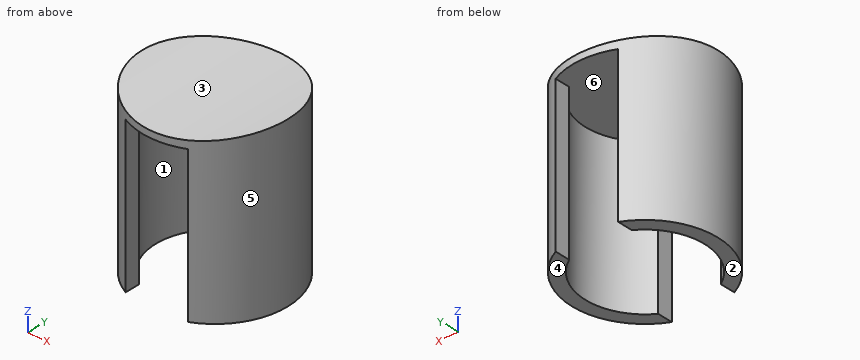
from build123d import *

# Parameters (mm, degrees)
F2_W     = 9.278574
F2_H     = 23.490808
F3_DEPTH = 22.747948
F4_R     = 65
F5_DEPTH = 12.5


with BuildPart() as f1:
    # F0 (on Front) → F1 (revolve)
    with BuildSketch(Plane.XZ):
        Polygon((10.8, -12.5), (10.8, 15.247948), (0, 15.247948), (0, 10.247948), (8.8, 10.247948), (8.8, -11.752052), (8.8, -12.5), align=None)
    revolve(axis=Axis((0, 0, 12.181249), (0, 0, 1)))

    # F2 (on face) → F3 (cut, through all)
    with BuildSketch(Plane(origin=(0, 0, -12.5), x_dir=(1, 0, 0), z_dir=(0, 0, -1))):
        Rectangle(F2_W, F2_H)
    extrude(amount=-F3_DEPTH, mode=Mode.SUBTRACT)

    # F4 (on Front) → F5 (cut, symmetric)
    with BuildSketch(Plane.XZ):
        with Locations((0, 76.247948)):
            Circle(F4_R)
    extrude(amount=F5_DEPTH, both=True, mode=Mode.SUBTRACT)


solid = f1.part
Can you work these out from the model? Positions are in its coordinate system, mm. Face numbers are marked on the shaded views. A direction names the side the tool comes from. Give positions to 0.01 mm unless a question says otherwise; leave off trailing zeros. Loops run counter-clockwise (first coordinate to the right, second up) from the corner with the lowest first, then second, coordinate; pieces in that order, holes last. Notation, with made-up numbers: (-16.75, 46.5) - (31.25, 46.5) arc R25 ccw to (31.25, 65.5) - close; hole circle Ø4 at (-27, 32). An arc over 180 degrees is marked (long way). One line per item, written item: value.
(1) If we section it at A-A, the plane z = -5: List the corners of the cut face in (x, y) for me.
Verdict:
outline: (-4.64, -9.75) - (-4.64, -7.48) arc R8.8 cw to (-4.64, 7.48) - (-4.64, 9.75) arc R10.8 ccw to start; (4.64, -9.75) arc R10.8 ccw to (4.64, 9.75) - (4.64, 7.48) arc R8.8 cw to (4.64, -7.48) - close
(2) If we section it at B-B, the plane y = 0: List the corners of the cut face in (x, z) for me.
Verdict:
outline: (-10.8, -12.5) - (-8.8, -12.5) - (-8.8, 10.25) - (8.8, 10.25) - (8.8, -12.5) - (10.8, -12.5) - (10.8, 12.15) arc R65 cw to (-10.8, 12.15) - close
(3) If we mould it in two halves opening along X, with no side actions, what happens to the marked faces 3, 4, 5 and 6? For each: released by +X, released by -X, zero draft, split by the parting line, or undercut.
Verdict:
face 3: undercut
face 4: zero draft
face 5: split by the parting line
face 6: undercut
(4) If we section it at C-C, the plane x = -5.5: List the corners of the cut face in (y, z) for me.
Verdict:
outline: (-9.29, -12.5) - (-6.87, -12.5) - (-6.87, 10.25) - (6.87, 10.25) - (6.87, -12.5) - (9.29, -12.5) - (9.29, 11.48) - (-9.29, 11.48) - close
(5) On a 3-axis mill with a long thin cutter (end or side, diameter ignored), from which of +Z, -Z, +X, -X, +Y, -Y can I reach the whole of each face in a straight line? I mean the marked faces 1 and 2. Say none if no direction works.
Verdict:
face 1: -Z
face 2: -Z, +X, -X, +Y, -Y
(6) I need wall thicknesses on line 1 along Z through (x, y) = (-1, -5.5); line 2 along X through (y, z) = (2.5, 4.5); line 3 along X through (y, z) = (-3, -1.75). Which ranges of each line are inside material? Lowest first, please.
Verdict:
line 1: 10.25 to 11.26
line 2: -10.51 to -8.44, 8.44 to 10.51
line 3: -10.37 to -8.27, 8.27 to 10.37
(7) I'm going to push flat-ended pins straight in: pin 1 (5.5 mm diameter, centred on x = 2.5, y = -5, fed in from -Z); pin 2 (6 mm diameter, centred on x = -8.5, z = -5.5, fed in from -Y); pin 3 (1.5 mm diameter, centred on x = -6.5, z = -3, fed in from +Y). Where does each tip first touch, or does it pass through?
Verdict:
pin 1: z = 10.25
pin 2: y = -9.29
pin 3: y = 9.14
(8) If we section it at D-D, the plane x = 0: List the corners of the cut face in (y, z) for me.
Verdict:
outline: (-10.8, 10.25) - (10.8, 10.25) - (10.8, 11.25) - (-10.8, 11.25) - close
